For this review, use the dimensioned drawing (mm, ordinates from the lowest corner) and the shaded views. A direction names the side the tool comes from. Coordinates: 2 decimals unless noted, no trailing zeros. Order: outer loops, then holes, each group sorted by start corner. A loop starts at its lowest first (then second) coordinate and runs counter-clockwise, first axis right, second up. Notation, with made-up numbers: M 65,42 L 88,42 A11 cw 88,54 Z; hole C -30.75,-6 d4. An arc over 180 degrees is marked long. Answer in a Markdown table with one row per item.
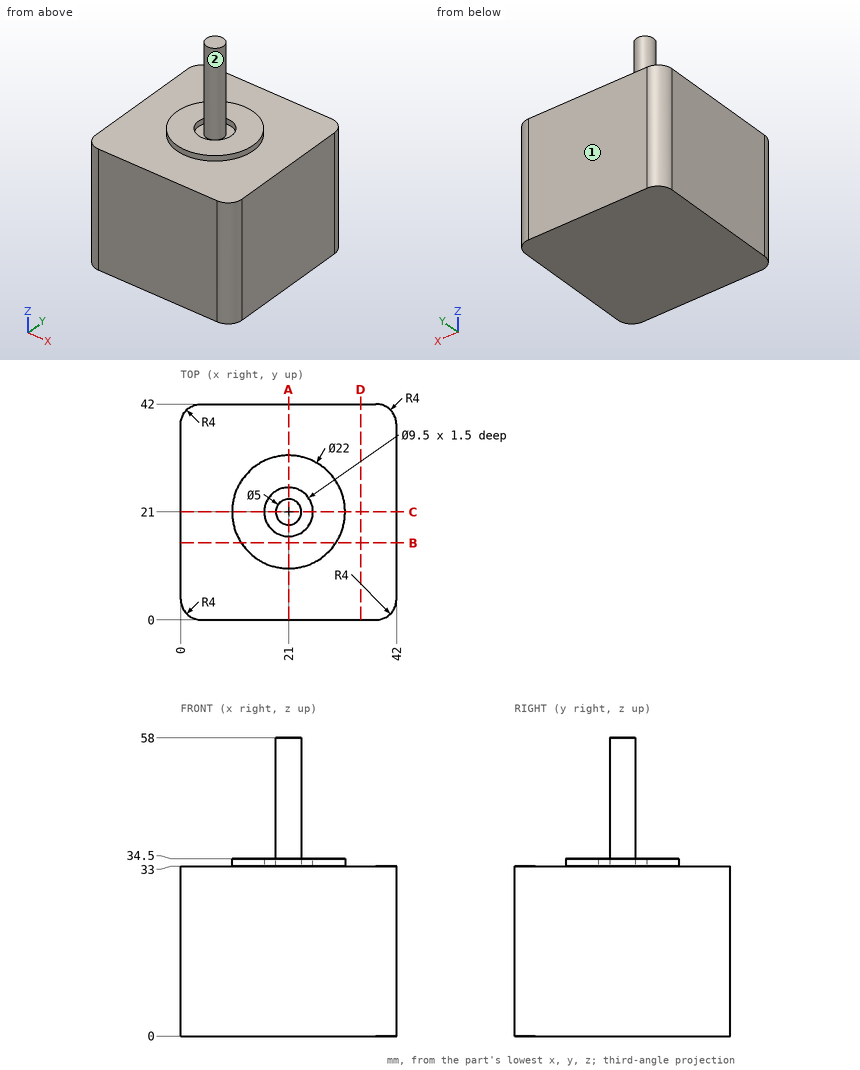
(1) Take a section at B-B (y = 15). Write out the cut boundary in (x, z).
Report:
| item | result |
|---|---|
| outline | M 0,0 L 42,0 L 42,33 L 30.22,33 L 30.22,34.5 L 11.78,34.5 L 11.78,33 L 0,33 Z |
(2) Take a section at A-A (x = 21). Write out the cut boundary in (y, z), then the cut area to 3 significant figures.
Report:
| item | result |
|---|---|
| outline | M 0,0 L 42,0 L 42,33 L 32,33 L 32,34.5 L 25.75,34.5 L 25.75,33 L 23.5,33 L 23.5,58 L 18.5,58 L 18.5,33 L 16.25,33 L 16.25,34.5 L 10,34.5 L 10,33 L 0,33 Z |
| area | 1,530 mm^2 |
(3) To check wall thickness, follow line 1 (Y direction, x = 21, z = 33.8); line 2 (Z direction, x = 34.5, y = 22.5); line 3 (Z direction, x = 28, y = 16). State the ranges of each line that lie inside material, in increasing order. Write a range as [from, to].
Report:
| item | result |
|---|---|
| line 1 | [10, 16.25], [18.5, 23.5], [25.75, 32] |
| line 2 | [0, 33] |
| line 3 | [0, 34.5] |
(4) Insertion check: P1, Ø2, axis at x = 18, y = 30.5, coming from the +Z side; P2, Ø8, axis at x = 31.5, y = 5, coming from the +Z side. Each pin has a flat end and moves straight along its axis. Give the tip position at first contact, or say it passes through.
Report:
| item | result |
|---|---|
| P1 | z = 34.5 |
| P2 | z = 33 |
(5) Machinability: for the marked faces 1 and 2, which of the approach directions +Z, -Z, +X, -X, +Y, -Y give a long, thin tool a straight path to every point of the face, cutting with its end or side? Answer none if there is none.
Report:
| item | result |
|---|---|
| face 1 | +Z, -Z, +X, -X, +Y |
| face 2 | +Z |
(6) Take a section at D-D (x = 35). Write out the cut boundary in (y, z), then the cut area to 3 significant figures.
Report:
| item | result |
|---|---|
| outline | M 0,0 L 42,0 L 42,33 L 0,33 Z |
| area | 1,390 mm^2 |
